Check sheet for the modelled part. Datum: model origin and axes. Units: mm. A direction names the side the tool comes from. Coordinates: 2 decimals unless noted, no trailing zeros. Write each loop counter-clockwise with the first axis right and the second up, starting at its lowest first coordinate (ties: lowest second). Pieces come first, ordered by that corner, then holes. Notation, with made-up numbers: M 45,59 L 93,59 A24 cw 93,71 Z; hole C 28.5,-25 d7. An arc over 180 degrees is marked long. Answer as CSV lines item,"result". Start each with the question number.
1) Section check C-C (x = 46). Record the cut outline in (y, z), and give its area (3 significant figures).
2) Access from +Z, -Z, +X, -X, +Y, -Y to the whole of each face (thin tool, end or side, straight path). Record for faces 3 (the flat face through (-4, -22, 3)), 4 (the flat face through (-3, -2, 7)), 5 (the flat face through (0, -15, 5)), 6 (the flat face through (55, 52.398, 1)).
3) Section check B-B (y = -20). Record the cut outline in (x, z), and give its area (3 significant figures).
4) Draft check along Y on faces 1 (the flat face through (-5, 29.2, 3.8)), 2 (the cylindrical face through (52.752, 55.099, 3.189)). Enter one of: +Y half, -Y half, draft (parallel to the pull), parting line (faces both ways), or undercut.
5) Material ranges on L1, parallel to Y at x = 55, z = 0.7; L2, parallel to Y at x = 5, z = 3.4; L3, parallel to Z at x = -1.3, y = 80, recorded low to high. Write a range as [from, to].
6) Section check D-D (y = 30). Record the cut outline in (x, z), and give its area (3 significant figures).
7) Section check A-A (x = 55). Record the cut outline in (y, z), and give its area (3 significant figures).
8) Go/stop test with flat-tipped pins: pin 1 Ø1.2 at (x, z) = (5, 1) entering from -Y; pin 2 Ø1.2 at (x, z) = (40, 2.5) entering from +Y; pin 3 Ø10 at (x, y) = (37.5, 60) entering from +Z; pin 4 Ø6 at (x, z) = (43, 7.5) entering from +Y. Record where each tip stops, or that it passes through.
from build123d import *

# Parameters (mm, degrees)
CYLINDER014_R             = 4
CYLINDER014_DEPTH         = 4
CYLINDER015_R             = 2.4
CYLINDER015_DEPTH         = 10
FUSION014_PLACEMENT_ANGLE = 90
CYLINDER016_R             = 4
CYLINDER016_DEPTH         = 4
CYLINDER017_R             = 2.4
CYLINDER017_DEPTH         = 10
FUSION015_PLACEMENT_ANGLE = 90
FUSION016_PLACEMENT_ANGLE = 270
BOX003_W                  = 5
BOX003_H                  = 64
BOX003_DEPTH              = 6
BOX002_W                  = 5
BOX002_H                  = 120
BOX002_DEPTH              = 10
CYLINDER021_R             = 22.5
CYLINDER021_DEPTH         = 10
CYLINDER018_R             = 2.25
CYLINDER018_DEPTH         = 10
EXTRUDE_DEPTH             = 2.4
CYLINDER019_R             = 2.25
CYLINDER019_DEPTH         = 10
CYLINDER020_R             = 2.25
CYLINDER020_DEPTH         = 10
BOX004_W                  = 60
BOX004_H                  = 60
BOX004_DEPTH              = 4


with BuildPart() as cylinder014:
    # Cylinder014 → Cylinder014 (new body)
    with BuildSketch(Plane.XY):
        Circle(CYLINDER014_R)
    extrude(amount=CYLINDER014_DEPTH)


with BuildPart() as fusion014:
    # Cylinder015 → Cylinder015 (new body)
    with BuildSketch(Plane.XY):
        Circle(CYLINDER015_R)
    extrude(amount=CYLINDER015_DEPTH)

    # Fusion014: union Cylinder014
    add(cylinder014.part)


with BuildPart() as fusion014_1:
    # Fusion014 placement: moved
    add(fusion014.part.moved(Location((-50, 0, 5))).rotate(Axis((-50, 0, 5), (1, 0, 0)), FUSION014_PLACEMENT_ANGLE))


with BuildPart() as cylinder016:
    # Cylinder016 → Cylinder016 (new body)
    with BuildSketch(Plane.XY):
        Circle(CYLINDER016_R)
    extrude(amount=CYLINDER016_DEPTH)


with BuildPart() as fusion016:
    # Cylinder017 → Cylinder017 (new body)
    with BuildSketch(Plane.XY):
        Circle(CYLINDER017_R)
    extrude(amount=CYLINDER017_DEPTH)

    # Fusion015: union Cylinder016
    add(cylinder016.part)


with BuildPart() as fusion016_1:
    # Fusion015 placement: moved
    add(fusion016.part.moved(Location((50, 0, 5))).rotate(Axis((50, 0, 5), (1, 0, 0)), FUSION015_PLACEMENT_ANGLE))

    # Fusion016: union Fusion014
    add(fusion014_1.part)


with BuildPart() as fusion016_2:
    # Fusion016 placement: moved
    add(fusion016_1.part.moved(Location((0, 30, 0))).rotate(Axis((0, 30, 0), (0, 0, 1)), FUSION016_PLACEMENT_ANGLE))


with BuildPart() as cube003:
    # Box003 → Box003 (new body)
    with BuildSketch(Plane(origin=(-5, -2, 4), x_dir=(1, 0, 0), z_dir=(0, 0, 1))):
        with Locations((2.5, 32)):
            Rectangle(BOX003_W, BOX003_H)
    extrude(amount=BOX003_DEPTH)


with BuildPart() as cut004:
    # Box002 → Box002 (new body)
    with BuildSketch(Plane(origin=(-5, -30, 0), x_dir=(1, 0, 0), z_dir=(0, 0, 1))):
        with Locations((2.5, 60)):
            Rectangle(BOX002_W, BOX002_H)
    extrude(amount=BOX002_DEPTH)

    # Cut003: cut Cube003
    add(cube003.part, mode=Mode.SUBTRACT)

    # Cut004: cut Fusion016
    add(fusion016_2.part, mode=Mode.SUBTRACT)


with BuildPart() as sphere001:
    # Sphere001 → Sphere001 (revolve)
    with BuildSketch(Plane(origin=(5, 55, 5), x_dir=(1, 0, 0), z_dir=(0, -1, 0))):
        with BuildLine():
            ThreePointArc((0, -4), (4, 0), (0, 4))
            Line((0, 4), (0, -4))
        make_face()
    revolve(axis=Axis((5, 55, 5), (0, 0, 1)))


with BuildPart() as cylinder021:
    # Cylinder021 → Cylinder021 (new body)
    with BuildSketch(Plane(origin=(30, 30, 0), x_dir=(1, 0, 0), z_dir=(0, 0, 1))):
        Circle(CYLINDER021_R)
    extrude(amount=CYLINDER021_DEPTH)


with BuildPart() as cylinder018:
    # Cylinder018 → Cylinder018 (new body)
    with BuildSketch(Plane(origin=(5, 5, 0), x_dir=(1, 0, 0), z_dir=(0, 0, 1))):
        Circle(CYLINDER018_R)
    extrude(amount=CYLINDER018_DEPTH)


with BuildPart() as din934_m007:
    # Sketch → Extrude (new body)
    with BuildSketch(Plane.XY):
        Polygon((-3.005, 0), (-1.5025, -2.602406), (1.5025, -2.602406), (3.005, 0), (1.5025, 2.602406), (-1.5025, 2.602406), align=None)
    extrude(amount=EXTRUDE_DEPTH)


with BuildPart() as fusion018:
    # Link004 base: copy of DIN934_M007
    add(din934_m007.part)


with BuildPart() as fusion018_1:
    # Link004 placement: moved
    add(fusion018.part.moved(Location((5, 5, 0))))

    # Fusion018: union Cylinder018
    add(cylinder018.part)


with BuildPart() as cylinder019:
    # Cylinder019 → Cylinder019 (new body)
    with BuildSketch(Plane(origin=(55, 5, -3), x_dir=(1, 0, 0), z_dir=(0, 0, 1))):
        Circle(CYLINDER019_R)
    extrude(amount=CYLINDER019_DEPTH)


with BuildPart() as fusion019:
    # Link005 base: copy of DIN934_M007
    add(din934_m007.part)


with BuildPart() as fusion019_1:
    # Link005 placement: moved
    add(fusion019.part.moved(Location((55, 5, 0))))

    # Fusion019: union Cylinder019
    add(cylinder019.part)


with BuildPart() as fusion019_2:
    # Fusion019 placement: moved
    add(fusion019_1.part.moved(Location((0, 0, 2))))


with BuildPart() as cylinder020:
    # Cylinder020 → Cylinder020 (new body)
    with BuildSketch(Plane(origin=(55, 55, 0), x_dir=(1, 0, 0), z_dir=(0, 0, 1))):
        Circle(CYLINDER020_R)
    extrude(amount=CYLINDER020_DEPTH)


with BuildPart() as compound002:
    # Link003 base: copy of DIN934_M007
    add(din934_m007.part)


with BuildPart() as compound002_1:
    # Link003 placement: moved
    add(compound002.part.moved(Location((55, 55, 0))))

    # Fusion017: union Cylinder020
    add(cylinder020.part)

    # Compound002: union Fusion018, Fusion019
    add(fusion018_1.part)
    add(fusion019_2.part)


with BuildPart() as obj1:
    # Box004 → Box004 (new body)
    with BuildSketch(Plane.XY):
        with Locations((30, 30)):
            Rectangle(BOX004_W, BOX004_H)
    extrude(amount=BOX004_DEPTH)

    # Cut005: cut Compound002
    add(compound002_1.part, mode=Mode.SUBTRACT)

    # Cut006: cut Cylinder021
    add(cylinder021.part, mode=Mode.SUBTRACT)

    # Fusion020: union Sphere001
    add(sphere001.part)

    # Fusion021: union Cut004
    add(cut004.part)


solid = obj1.part
Results found:
1,outline,"M 0,0 L 14.18,0 L 14.18,4 L 0,4 Z; M 45.82,0 L 60,0 L 60,4 L 45.82,4 Z"
1,area,"113 mm2"
2,face 3,"+X"
2,face 4,"+Z, +X, -X"
2,face 5,"+Z, -Z, +X, -Y"
2,face 6,"-Z"
3,outline,"M -5,0 L 0,0 L 0,1 L -4,1 L -4,2.6 L -5,2.6 Z; M -5,7.4 L -4,7.4 L -4,9 L 0,9 L 0,10 L -5,10 Z"
3,area,"13.2 mm2"
4,face 1,"draft"
4,face 2,"undercut"
5,L1,"y = [0, 2.75], [7.25, 52.4], [57.6, 60]"
5,L2,"y = [0, 2.75], [7.25, 60]"
5,L3,"z = [0, 1], [9, 10]"
6,outline,"M -5,0 L 7.5,0 L 7.5,4 L -5,4 Z; M 52.5,0 L 60,0 L 60,4 L 52.5,4 Z"
6,area,"80.0 mm2"
7,outline,"M 0,0 L 2.75,0 L 2.75,2 L 2.4,2 L 2.4,4 L 0,4 Z; M 7.25,0 L 52.4,0 L 52.4,2.4 L 52.75,2.4 L 52.75,4 L 7.6,4 L 7.6,2 L 7.25,2 Z; M 57.25,2.4 L 57.6,2.4 L 57.6,0 L 60,0 L 60,4 L 57.25,4 Z"
7,area,"201 mm2"
8,pin 1,"stops at y = 0"
8,pin 2,"stops at y = 60"
8,pin 3,"stops at z = 4"
8,pin 4,"passes through"
